Design review of the part built by this model. Coordinates are the model's own, in mm. A direction names the side the tool comes from. Round coordinates to 2 decimals unless told otherwise and drop trailing zeros. Order: outer loops, then holes, each group sorted by start corner. A loop starts at its lowest first (then second) coordinate and runs counter-clockwise, first axis right, second up. Notation, with made-up numbers: M 8,-10.75 L 55,-10.75 A19 ccw 55,-6.75 Z; hole C -24,-21.75 d5. An arc over 180 degrees is marked long. Write item = value, one per line. Start each with the question number.
```python
from build123d import *

# Parameters (mm, degrees)
F2_W     = 21
F2_H     = 15
F3_DEPTH = 10.5
F3_TAPER = -0.16


with BuildPart() as f1:
    # F0 (on Top) → F1 (revolve)
    with BuildSketch(Plane.XY):
        Polygon((5, 3.5), (0, 3.5), (0, 0), (5, 0), (5, 2.5), align=None)
        Polygon((12, 3.5), (5, 3.5), (5, 2.5), (16, 2.5), (16, 3.5), align=None)
        Polygon((12, 5.5), (12, 3.5), (16, 3.5), align=None)
    revolve(axis=Axis((2.5, 0, 0), (1, 0, 0)))

    # F2 (on Front) → F3 (cut, symmetric)
    with BuildSketch(Plane.XZ):
        with Locations((10.5, 9.5)):
            Rectangle(F2_W, F2_H)
        with Locations((10.5, -9.5)):
            Rectangle(F2_W, F2_H)
    extrude(amount=F3_DEPTH, both=True, taper=F3_TAPER, mode=Mode.SUBTRACT)

    # F4: F1 across plane


with BuildPart() as f1_1:
    add(f1.part)
    add(f1.part.mirror(Plane.YZ))


solid = f1_1.part
```
(1) Consider section A-A, the plane x = 7.5. Write out the cut boundary in (y, z), then the cut area to 3 significant figures.
(2) Consider section B-B, the plane x = 12.5. Write out the cut boundary in (y, z), then the cut area to 3 significant figures.
(3) For faces 1 (the face through (-10.6, 2.5, 0)), 2 (the face through (14.4, -4.3, 0)), 3 (the face through (5, 0, 0)), list the 3-axis set-ups (+Z, -Z, +X, -X, +Y, -Y) from which the entire face can be reached by the end or side of a thin tool; tool diameter is ignored.
(4) Insertion check: pin 1 (1 mm diameter, centred on y = -1.5, z = 0.5, fed in from +X); pin 2 (1.3 mm diameter, centred on y = 4.5, z = 1, fed in from +X); pin 3 (1 mm diameter, centred on x = -11, y = 4.5, fed in from +Z); pin 4 (5 mm diameter, centred on x = 2, y = -3.5, fed in from +Z). Each pin has a flat end and moves straight along its axis. Give the tip position at first contact, or say it passes through.
(5) Draft analysis for pull direction Z (two halves, no side actions). For faces 4 (the face through (-10.6, -2.5, 0)), 5 (the face through (-14.4, 4.3, 0)), 6 (the face through (16, 3, 0)), state which applies: pulls with the +Z half, pulls with the -Z half, needs draft (parallel to the pull), parting line crosses it, or undercut.
(6) Consider section D-D, the plane y = -1. Write out the cut boundary in (x, z).
(7) Consider section C-C, the plane x = -2.5. Write out the cut boundary in (y, z), then the cut area to 3 significant figures.
(8) For line 1 along Z through (x, y) = (7, 2); line 2 along Y through (x, z) = (0.5, 0.05); line 3 along X through (y, z) = (-3.75, -0.8), list the stretches that pass through material, from the lowest coordinate up. Write a range as [from, to].
Completed:
q1.outline = M -2.88,-1.99 L -1.51,-2 A2.5 cw -1.51,2 L -2.88,1.99 A3.5 ccw Z; M 1.51,-2 L 2.88,-1.99 A3.5 ccw 2.88,1.99 L 1.51,2 A2.5 cw Z
q1.area = 8.77 mm2
q2.outline = M -4.86,-1.99 L -1.51,-2 A2.5 cw -1.51,2 L -4.86,1.99 A5.25 ccw Z; M 1.51,-2 L 4.86,-1.99 A5.25 ccw 4.86,1.99 L 1.51,2 A2.5 cw Z
q2.area = 23.3 mm2
q3.face_1 = -X
q3.face_2 = +X, -Y
q3.face_3 = +X
q4.pin_1 = 5
q4.pin_2 = 15.08
q4.pin_3 = through
q4.pin_4 = 2
q5.face_4 = undercut
q5.face_5 = parting line crosses it
q5.face_6 = needs draft
q6.outline = M -5,-2 L 5,-2 L 5,2 L -5,2 Z
q7.outline = M -2.88,-1.99 L 0,-2 L 2.88,-1.99 A3.5 ccw 2.88,1.99 L 0,2 L -2.88,1.99 A3.5 ccw Z
q7.area = 26.3 mm2
q8.line_1 = [-1.99, -1.5], [1.5, 1.99]
q8.line_2 = [-3.5, 3.5]
q8.line_3 = [-15.33, -12], [12, 15.33]
